Source: CAD feature listing. Evaluate the final solid. Frame: model axes, mm. Face numbers are marked on the shaded views. A direction names the side the tool comes from. Round coordinates to 2 decimals unless told otherwise and drop trailing zeros. Loops run counter-clockwise (first coordinate to the right, second up) from the corner with the lowest first, then second, coordinate; pieces in that order, holes last. Notation, with made-up numbers: M -29,-6.5 L 15,-6.5 A33 ccw 15,23.5 Z; hole C 20.5,68.25 d2. An arc over 180 degrees is marked long. Write each question's results on one line, items separated by ' | '. Start each with the question number.
1. Section C-C on y = 28.5. Give the number of separate pieces and of enclosed holes in the cut face, and give its area (3 significant figures).
2. Draft query along X for the marked faces 3, 4 and 5. Return one class per face: released by +X, released by -X, zero draft, split by the parting line, or undercut.
3. Section A-A on x = 53. Output: boundary loops of the cut face in (y, z), and give its area (3 significant figures).
4. Section B-B on z = -21.5. Output: boundary loops of the cut face in (x, y), and give its area (3 significant figures).
5. Set-up query: the marked faces 1 and 2. Return all of +Z, -Z, +X, -X, +Y, -Y with unobstructed straight access to the full face (end or side cutting, diameter ignored); none if empty.
6. Ray query, line 1 (X direction, y = 5, z = -17); line 2 (Z direction, x = 24, y = 48); line 3 (X direction, y = 12, z = -34). Return the intervals inside material, ascending.
from build123d import *

# Parameters (mm, degrees)
SKETCH2_W           = 60
SKETCH2_H           = 60
BOSS_EXTRUDE2_DEPTH = 80
CUT_EXTRUDE1_DEPTH  = 80
SKETCH4_R           = 7
BOSS_EXTRUDE3_DEPTH = 80
SKETCH5_W           = 2
SKETCH5_H           = 19.255437353
SKETCH5_W_2         = 19.265898102
SKETCH5_H_2         = 2
CUT_EXTRUDE2_DEPTH  = 80


with BuildPart() as part:
    # Sketch2 → Boss-Extrude2 (new body)
    with BuildSketch(Plane(origin=(0, 0, 0), x_dir=(1, 0, 0), z_dir=(0, 1, 0))):
        with Locations((30, 30)):
            Rectangle(SKETCH2_W, SKETCH2_H)
    extrude(amount=BOSS_EXTRUDE2_DEPTH)

    # Sketch3 → Cut-Extrude1 (cut)
    with BuildSketch(Plane(origin=(0, 80, 0), x_dir=(1, 0, 0), z_dir=(0, 1, 0))):
        with BuildLine():
            Line((26, 55), (15, 55))
            ThreePointArc((15, 55), (7.928932188, 52.071067812), (5, 45))
            Line((5, 45), (5, 34))
            Line((5, 34), (26, 34))
            Line((26, 34), (26, 55))
        make_face()
        with BuildLine():
            Line((45, 55), (34, 55))
            Line((34, 55), (34, 34))
            Line((34, 34), (55, 34))
            Line((55, 34), (55, 45))
            ThreePointArc((55, 45), (52.071067812, 52.071067812), (45, 55))
        make_face()
        with BuildLine():
            Line((26, 26), (5, 26))
            Line((5, 26), (5, 15))
            ThreePointArc((5, 15), (7.928932188, 7.928932188), (15, 5))
            Line((15, 5), (26, 5))
            Line((26, 5), (26, 26))
        make_face()
        with BuildLine():
            Line((55, 15), (55, 26))
            Line((55, 26), (34, 26))
            Line((34, 26), (34, 5))
            Line((34, 5), (45, 5))
            ThreePointArc((45, 5), (52.071067812, 7.928932188), (55, 15))
        make_face()
    extrude(amount=-CUT_EXTRUDE1_DEPTH, mode=Mode.SUBTRACT)

    # Sketch4 → Boss-Extrude3 (add)
    with BuildSketch(Plane.XZ):
        with Locations((30, -30)):
            Circle(SKETCH4_R)
    extrude(amount=-BOSS_EXTRUDE3_DEPTH)

    # Sketch5 → Cut-Extrude2 (cut)
    with BuildSketch(Plane.XZ):
        with Locations((27, -14.627718677)):
            Rectangle(SKETCH5_W, SKETCH5_H)
        with Locations((33, -14.627718677)):
            Rectangle(SKETCH5_W, SKETCH5_H)
        with Locations((45.367050949, -27)):
            Rectangle(SKETCH5_W_2, SKETCH5_H_2)
        with Locations((45.367050949, -33)):
            Rectangle(SKETCH5_W_2, SKETCH5_H_2)
        with Locations((33, -45.372281324)):
            Rectangle(SKETCH5_W, SKETCH5_H)
        with Locations((27, -45.372281324)):
            Rectangle(SKETCH5_W, SKETCH5_H)
        with Locations((14.632949051, -33)):
            Rectangle(SKETCH5_W_2, SKETCH5_H_2)
        with Locations((14.632949051, -27)):
            Rectangle(SKETCH5_W_2, SKETCH5_H_2)
    extrude(amount=-CUT_EXTRUDE2_DEPTH, mode=Mode.SUBTRACT)


solid = part.part
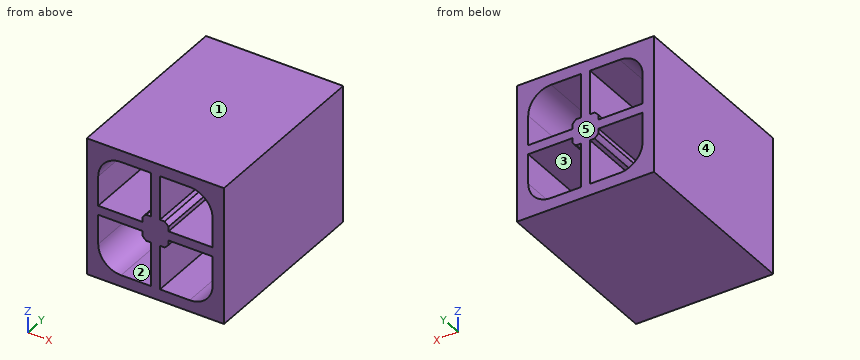
Taken from the geometry:
1) separate pieces: 1 | enclosed holes: 4 | area: 1,620 mm^2
2) face 3: undercut | face 4: released by -X | face 5: zero draft
3) outline: M 0,-60 L 80,-60 L 80,-51 L 0,-51 Z; M 0,-32 L 80,-32 L 80,-28 L 0,-28 Z; M 0,-9 L 80,-9 L 80,0 L 0,0 Z | area: 1,760 mm^2
4) outline: M 0,0 L 5,0 L 5,80 L 0,80 Z; M 28,0 L 32,0 L 32,80 L 28,80 Z; M 55,0 L 60,0 L 60,80 L 55,80 Z | area: 1,120 mm^2
5) face 1: +Z, +X, -X, +Y, -Y | face 2: +Y, -Y
6) line 1: 0 to 5, 28 to 32, 55 to 60 | line 2: -60 to -55, -32 to -28, -5 to 0 | line 3: 0 to 5, 24.27 to 35.73, 55 to 60
